```python
from build123d import *

# Parameters (mm, degrees)
F1_DEPTH  = 50.8
F2_W      = 19.05
F2_H      = 76.2
F3_DEPTH  = 838.2
F4_W      = 355.6
F4_H      = 76.2
F5_DEPTH  = 19.05
F6_W      = 44.45
F6_H      = 482.6
F7_DEPTH  = 19.05
F9_W      = 76.2
F9_H      = 19.05
F10_DEPTH = 1156.976414305
F8_W      = 292.7382071525
F8_H      = 19.05
F11_DEPTH = 76.2
F12_W     = 19.05
F12_H     = 203.2
F13_DEPTH = 76.2
F14_W     = 3.175
F14_H     = 203.2
F15_DEPTH = 431.8
F16_W     = 355.6
F16_H     = 76.2
F16_H_2   = 52.435785675
F17_DEPTH = 19.05
F20_W     = 19.05
F20_H     = 19.05
F22_W     = 533.4
F22_H     = 19.05
F22_W_2   = 292.7382071525
F23_DEPTH = 76.2
F25_DEPTH = 3.175


with BuildPart() as f1:
    # F0 (on Top) → F1 (new body)
    with BuildSketch(Plane.XY):
        Polygon((617.4126458168, 48.7991196131), (-703.3873541832, 48.7991196131), (-703.3873541832, -333.4772946919), (-577.6637684882, -459.2008803869), (617.4126458168, -459.2008803869), align=None)
    extrude(amount=F1_DEPTH)

    # F2 (on face) → F3 (join)
    with BuildSketch(Plane(origin=(0, 0, 0), x_dir=(1, 0, 0), z_dir=(0, 0, -1))):
        with Locations((607.8876458168, 421.1008803869)):
            Rectangle(F2_W, F2_H)
        with Locations((607.8876458168, -10.6991196131)):
            Rectangle(F2_W, F2_H)
        with Locations((-568.1387684882, 421.1008803869)):
            Rectangle(F2_W, F2_H)
        with Locations((-568.1387684882, -10.6991196131)):
            Rectangle(F2_W, F2_H)
    extrude(amount=F3_DEPTH)

    # F4 (on face) → F5 (join)
    with BuildSketch(Plane(origin=(-577.6637684882, 0, 0), x_dir=(0, -1, 0), z_dir=(-1, 0, 0))):
        with Locations((205.2008803869, -241.3)):
            Rectangle(F4_W, F4_H)
        with Locations((205.2008803869, -800.1)):
            Rectangle(F4_W, F4_H)
    extrude(amount=-F5_DEPTH)

    # F6 (on face) → F7 (join, through all)
    with BuildSketch(Plane(origin=(-577.6637684882, 0, 0), x_dir=(0, -1, 0), z_dir=(-1, 0, 0))):
        with Locations((81.3758803869, -520.7)):
            Rectangle(F6_W, F6_H)
        with Locations((163.9258803869, -520.7)):
            Rectangle(F6_W, F6_H)
        with Locations((246.4758803869, -520.7)):
            Rectangle(F6_W, F6_H)
        with Locations((329.0258803869, -520.7)):
            Rectangle(F6_W, F6_H)
    extrude(amount=-F7_DEPTH)

    # F9 (on face) → F10 (join, through all)
    with BuildSketch(Plane.YZ.offset(-558.6137684882)):
        with Locations((10.6991196131, -212.725)):
            Rectangle(F9_W, F9_H)
    extrude(amount=F10_DEPTH)

    # F8 (on face) → F11 (join)
    with BuildSketch(Plane.XZ.offset(459.2008803869)):
        Polygon((-246.8255613357, 0), (-265.8755613357, 0), (-265.8755613357, -203.2), (-265.8755613357, -222.25), (-246.8255613357, -222.25), align=None)
        with Locations((-412.244664912, -212.725)):
            Rectangle(F8_W, F8_H)
        Polygon((305.6244386643, 0), (286.5744386643, 0), (286.5744386643, -222.25), (305.6244386643, -222.25), (305.6244386643, -203.2), align=None)
        with Locations((451.9935422405, -212.725)):
            Rectangle(F8_W, F8_H)
    extrude(amount=-F11_DEPTH)

    # F12 (on face) → F13 (join)
    with BuildSketch(Plane(origin=(0, 48.7991196131, 0), x_dir=(-1, 0, 0), z_dir=(0, 1, 0))):
        with Locations((-296.0994386643, -101.6)):
            Rectangle(F12_W, F12_H)
        with Locations((256.3505613357, -101.6)):
            Rectangle(F12_W, F12_H)
    extrude(amount=-F13_DEPTH)

    # F14 (on face) → F15 (join, through all)
    with BuildSketch(Plane.XZ.offset(459.2008803869)):
        with Locations((-568.1387684882, -101.6)):
            Rectangle(F14_W, F14_H)
        with Locations((-256.3823113357, -101.6)):
            Rectangle(F14_W, F14_H)
        with Locations((296.0994386643, -101.6)):
            Rectangle(F14_W, F14_H)
        with Locations((607.8876458168, -101.6)):
            Rectangle(F14_W, F14_H)
    extrude(amount=-F15_DEPTH)

    # F16 (on face) → F17 (join)
    with BuildSketch(Plane.YZ.offset(617.4126458168)):
        with Locations((-205.2008803869, -241.3)):
            Rectangle(F16_W, F16_H)
        with Locations((-205.2008803869, -481.7821071625)):
            Rectangle(F16_W, F16_H_2)
    extrude(amount=-F17_DEPTH)

    # F21: sweep along a path in F19
    with BuildLine(Plane.XZ.offset(408.4008803869)) as f21_path:
        Line((-145.2255613357, 0), (-145.2255613357, -12.7))
        ThreePointArc((-145.2255613357, -12.7), (-126.6268419411, -57.6012806053), (-81.7255613357, -76.2))
        Line((-81.7255613357, -76.2), (121.4744386643, -76.2))
        ThreePointArc((121.4744386643, -76.2), (166.3757192696, -57.6012806053), (184.9744386643, -12.7))
        Line((184.9744386643, -12.7), (184.9744386643, 0))
    # F20 (on face) → F21 (sweep)
    with BuildSketch(Plane(origin=(0, 0, 0), x_dir=(1, 0, 0), z_dir=(0, 0, -1))):
        with Locations((-156.0781598091, 421.7912954004)):
            Rectangle(F20_W, F20_H)
    sweep(path=f21_path.line)

    # F22 (on face) → F23 (join)
    with BuildSketch(Plane.XZ.offset(459.2008803869)):
        Polygon((-246.8255613357, -488.95), (-246.8255613357, -222.25), (-265.8755613357, -222.25), (-265.8755613357, -488.95), (-265.8755613357, -508), (-246.8255613357, -508), align=None)
        with Locations((19.8744386643, -498.475)):
            Rectangle(F22_W, F22_H)
        with Locations((-412.244664912, -498.475)):
            Rectangle(F22_W_2, F22_H)
        Polygon((286.5744386643, -222.25), (286.5744386643, -488.95), (286.5744386643, -508), (305.6244386643, -508), (305.6244386643, -488.95), (305.6244386643, -222.25), align=None)
        with Locations((451.9935422405, -498.475)):
            Rectangle(F22_W_2, F22_H)
    extrude(amount=-F23_DEPTH)

    # F24 (on offset) → F25 (join)
    with BuildSketch(Plane.XZ.offset(408.4008803869)):
        Polygon((-558.6137684882, -222.25), (-558.6137684882, -488.95), (598.3626458168, -488.95), (598.3626458168, -222.25), (286.5744386643, -222.25), (286.5744386643, 0), (-246.8255613357, 0), (-246.8255613357, -222.25), align=None)
    extrude(amount=F25_DEPTH)


solid = f1.part
```
CAD build for the part. Positions are in the model's coordinates, mm. A direction names the side the tool comes from. Give positions to 0.01 mm unless a question says otherwise; leave off trailing zeros. Write each loop counter-clockwise with the first axis right and the second up, starting at its lowest first coordinate (ties: lowest second). Pieces come first, ordered by that corner, then holes. Notation, with made-up numbers: M 52.5,-26.5 L 57.5,-26.5 A27 cw 57.5,4.5 Z; hole C -3.75,-29.5 d5. An arc over 180 degrees is marked long. Return JSON: item names as keys, results as strings. Group by question number.
(1) Flat gauge pins, fed straight in: pin 1 Ø1.5 at (y, z) = (-387, -454.5) entering from -X; pin 2 Ø9.5 at (x, y) = (17.5, -422.5) entering from -Z; pin 3 Ø4 at (x, y) = (-24, -94.5) entering from -Z. Where does each tip first touch, or does it go through?
(2) Band-saw the part on B-B (x = -45). Give the cut face in (y, z).
(3) Band-saw the part on A-A (z = -699.5). State how many separate pieces and enclosed holes the cut face has, and give its area (3 significant figures).
(4) Drill centre lines: L1, parallel to X at y = -411, z = -124.5; L2, parallel to X at y = -238.5, z = -159.5; L3, parallel to Y at x = -264, z = -133.5. Where is each one in solid material? Low to high. Write a range as [from, to].
(5) 3-axis set-ups, long thin cutter, end or side, ignore diameter. For faces 5 (the face through (-414, -408.401, -354)), 6 (the face through (286.574, -436, -241)), 7 (the face through (-257.97, -208, -103)): which of +Z, -Z, +X, -X, +Y, -Y reach the whole face in a straight line?
(6) Mould opens along Y. For faces 1 (the face through (450, -411.576, -354)), 2 (the face through (12, 10, -222.25)), 3 (the face through (294.512, -208, -103)), 4 (the face through (450, -408.401, -354)) say: pulls with the +Y half, pulls with the -Y half, needs draft (parallel to the pull), parting line crosses it, or undercut.
(7) Band-saw the part on D-D (x = -363.5). Give the cut face in (y, z), and give its area (3 significant figures).
Entries:
{
 "1": {"pin 1": "stops at x = -577.66", "pin 2": "stops at z = -508", "pin 3": "stops at z = 0"},
 "2": {"outline": "M -459.2,-508 L -383,-508 L -383,-488.95 L -408.4,-488.95 L -408.4,0 L 48.8,0 L 48.8,50.8 L -459.2,50.8 L -459.2,0 L -411.58,0 L -411.58,-488.95 L -459.2,-488.95 Z; M -431.32,-96.58 L -412.27,-96.58 L -412.27,-77.53 L -431.32,-77.53 Z; M -27.4,-222.25 L 48.8,-222.25 L 48.8,-203.2 L -27.4,-203.2 Z"},
 "3": {"separate pieces": "8", "enclosed holes": "0", "area": "9,190 mm^2"},
 "4": {"L1": "x = [-577.66, -558.61], [-265.88, 305.62], [598.36, 617.41]", "L2": "x = [-569.73, -566.55], [-257.97, -254.79], [294.51, 297.69], [606.3, 609.48]", "L3": "y = [-459.2, -383], [-27.4, 48.8]"},
 "5": {"face 5": "+Y", "face 6": "-Y", "face 7": "-Z"},
 "6": {"face 1": "pulls with the -Y half", "face 2": "needs draft", "face 3": "undercut", "face 4": "pulls with the +Y half"},
 "7": {"outline": "M -459.2,-508 L -383,-508 L -383,-488.95 L -408.4,-488.95 L -408.4,-222.25 L -383,-222.25 L -383,-203.2 L -459.2,-203.2 L -459.2,-222.25 L -411.58,-222.25 L -411.58,-488.95 L -459.2,-488.95 Z; M -459.2,0 L 48.8,0 L 48.8,50.8 L -459.2,50.8 Z; M -27.4,-222.25 L 48.8,-222.25 L 48.8,-203.2 L -27.4,-203.2 Z", "area": "31,000 mm^2"}
}
